```python
from build123d import *

# Parameters (mm, degrees)
SKETCH1_W                       = 160
SKETCH1_H                       = 36
BOSS_EXTRUDE1_DEPTH             = 3
SKETCH3_W                       = 160
SKETCH3_H                       = 36
SKETCH3_W_2                     = 156
SKETCH3_H_2                     = 32
BOSS_EXTRUDE3_DEPTH             = 20
SKETCH4_W                       = 2
SKETCH4_H                       = 1
CUT_EXTRUDE1_DEPTH              = 20
SKETCH5_R                       = 4.5
BOSS_EXTRUDE4_DEPTH             = 20
F_5_0MM_DOWEL_HOLE1_D           = 5
F_5_0MM_DOWEL_HOLE1_DEPTH       = 4.6
F_5_0MM_DOWEL_HOLE1_CSINK_D     = 6
F_5_0MM_DOWEL_HOLE1_CSINK_ANGLE = 90
FILLET3_R                       = 3
M5_CLEARANCE_HOLE2_D            = 5.5
FILLET4_R                       = 1
M5_CLEARANCE_HOLE3_D            = 5.5
M5_CLEARANCE_HOLE3_DEPTH        = 10
M5_CLEARANCE_HOLE3_TIP          = 1.652366702


with BuildPart() as part:
    # Sketch1 → Boss-Extrude1 (new body)
    with BuildSketch(Plane.XY):
        Rectangle(SKETCH1_W, SKETCH1_H)
    extrude(amount=BOSS_EXTRUDE1_DEPTH)

    # Sketch3 → Boss-Extrude3 (add)
    with BuildSketch(Plane.XY.offset(3)):
        Rectangle(SKETCH3_W, SKETCH3_H)
        Rectangle(SKETCH3_W_2, SKETCH3_H_2, mode=Mode.SUBTRACT)
    extrude(amount=BOSS_EXTRUDE3_DEPTH)

    # Sketch4 → Cut-Extrude1 (cut)
    with BuildSketch(Plane.XY.offset(23)):
        with Locations((79, 0)):
            Rectangle(SKETCH4_W, SKETCH4_H)
    cut_extrude1 = extrude(amount=-CUT_EXTRUDE1_DEPTH, mode=Mode.SUBTRACT)

    # Sketch5 → Boss-Extrude4 (add)
    with BuildSketch(Plane.XY.offset(3)):
        with Locations((75, 13)):
            Circle(SKETCH5_R)
        with Locations((75, -13)):
            Circle(SKETCH5_R)
    boss_extrude4 = extrude(amount=BOSS_EXTRUDE4_DEPTH)

    # Ø5.0mm Dowel Hole1
    with Locations(Plane.XY.offset(23)):
        with Locations((75, 13), (75, -13)):
            f_5_0mm_dowel_hole1 = CounterSinkHole(F_5_0MM_DOWEL_HOLE1_D / 2, F_5_0MM_DOWEL_HOLE1_CSINK_D / 2, depth=F_5_0MM_DOWEL_HOLE1_DEPTH, counter_sink_angle=F_5_0MM_DOWEL_HOLE1_CSINK_ANGLE)

    # Fillet3
    fillet3_edges = [part.edges().sort_by_distance(p)[0] for p in [
        (-80, 18, 11.5),
        (80, 18, 11.5),
        (80, -18, 11.5),
        (-80, -18, 11.5),
    ]]
    fillet(fillet3_edges, radius=FILLET3_R)

    # M5 Clearance Hole2 (through all)
    with Locations(Plane(origin=(0, 0, 0), x_dir=(-1, 0, 0), z_dir=(0, 0, -1))):
        with Locations((-70, 0), (70, 0)):
            m5_clearance_hole2 = Hole(M5_CLEARANCE_HOLE2_D / 2)

    # Mirror2: Cut-Extrude1, Boss-Extrude4, Ø5.0mm Dowel Hole1, M5 Clearance Hole2 across plane
    add(cut_extrude1.mirror(Plane(origin=(0, 0, 0), x_dir=(0, 0, 1), z_dir=(1, 0, 0))), mode=Mode.SUBTRACT)
    add(boss_extrude4.mirror(Plane(origin=(0, 0, 0), x_dir=(0, 0, 1), z_dir=(1, 0, 0))))
    add(f_5_0mm_dowel_hole1.mirror(Plane(origin=(0, 0, 0), x_dir=(0, 0, 1), z_dir=(1, 0, 0))), mode=Mode.SUBTRACT)
    add(m5_clearance_hole2.mirror(Plane(origin=(0, 0, 0), x_dir=(0, 0, 1), z_dir=(1, 0, 0))), mode=Mode.SUBTRACT)

    # Fillet4
    fillet4_edges = [part.edges().sort_by_distance(p)[0] for p in [
        (-78, -9.645898034, 13),
        (-78, -0.5, 13),
        (-80, -0.5, 13),
        (-80, 0.5, 13),
        (-78, 0.5, 13),
        (-78, 9.645898034, 13),
        (-71.645898034, 16, 13),
        (71.645898034, 16, 13),
        (78, 0.5, 13),
        (80, 0.5, 13),
        (80, -0.5, 13),
        (78, -0.5, 13),
        (78, -9.645898034, 13),
        (71.645898034, -16, 13),
        (-71.645898034, -16, 13),
        (78, 9.645898034, 13),
    ]]
    fillet(fillet4_edges, radius=FILLET4_R - 0.0001)  # a hair under: the kernel refuses the full size

    # M5 Clearance Hole3
    with Locations(Plane(origin=(80, 0, 0), x_dir=(0, 0, -1), z_dir=(1, 0, 0))):
        with Locations((-21.351359234, 0)):
            Hole(M5_CLEARANCE_HOLE3_D / 2, depth=M5_CLEARANCE_HOLE3_DEPTH)
            with Locations((0, 0, -(M5_CLEARANCE_HOLE3_DEPTH + M5_CLEARANCE_HOLE3_TIP / 2))):  # 118° drill point
                Cone(0, M5_CLEARANCE_HOLE3_D / 2, M5_CLEARANCE_HOLE3_TIP, mode=Mode.SUBTRACT)


solid = part.part
```
Verification items for the finished model (mm, model axes). A direction names the side the tool comes from. Round coordinates to 2 decimals unless told otherwise and drop trailing zeros. Order: outer loops, then holes, each group sorted by start corner. A loop starts at its lowest first (then second) coordinate and runs counter-clockwise, first axis right, second up. Notation, with made-up numbers: (-33.75, 66.25) -> (-12.75, 66.25) arc R20 cw to (-12.75, 70.25) -> close; hole circle Ø5 at (69.25, -30.5). An arc over 180 degrees is marked (long way). Put each result on its own line as item: value. Start each with the question number.
(1) Depth check by flat-ended pin: pin 1 Ø4.5 at (x, y) = (-70, 0) entering from -Z; pin 2 Ø2.5 at (x, y) = (75, -13.5) entering from +Z; pin 3 Ø1 at (x, y) = (12.5, -3.5) entering from +Z; pin 4 Ø2.5 at (x, y) = (74, 14) entering from +Z. Enter the tip coordinate at first touch or a pass-through.
(2) Material ranges on line 1 along X through (y, z) = (-13, 20.85); line 2 along X through (y, z) = (0, 1.6); line 3 along Y through (x, z) = (75, 21.15), recorded low to high.
(3) Section check A-A (x = -12.5). Enter the section's corners in (y, z).
(4) Tool access check on faces 1 (the face through (-80, -4, 11)), 2 (the face through (-71.87, -9.767, 12.86)). Record the directions out of +Z, -Z, +X, -X, +Y, -Y that give a thin tool (end or side, any length) a straight path to the whole face; none if there is none.
(5) Draft check along X on faces 3 (the face through (-78, -5, 13)), 4 (the face through (80, -4, 11)), 5 (the face through (-1, -18, 11)), 6 (the face through (78, -5, 13)). Enter one of: +X half, -X half, draft (parallel to the pull), parting line (faces both ways), or undercut.
(6) Section check C-C (x = 75). Enter the section's corners in (y, z), then the cut area to 4 significant figures.
(7) Section check B-B (y = -6). Enter the section's corners in (x, z).
Completed:
1. pin 1: passes through
1. pin 2: stops at z = 18.4
1. pin 3: stops at z = 3
1. pin 4: stops at z = 22.66
2. line 1: x = -80 to -77.5, -72.5 to -70.5, 70.5 to 72.5, 77.5 to 80
2. line 2: x = -80 to -72.75, -67.25 to 67.25, 72.75 to 80
2. line 3: y = -18 to -15.5, -10.5 to -8.5, 8.5 to 10.5, 15.5 to 18
3. outline: (-18, 0) -> (18, 0) -> (18, 23) -> (16, 23) -> (16, 3) -> (-16, 3) -> (-16, 23) -> (-18, 23) -> close
4. face 1: +Z, -Z, -X, +Y, -Y
4. face 2: +Z
5. face 3: undercut
5. face 4: +X half
5. face 5: draft
5. face 6: undercut
6. outline: (-18, 0) -> (18, 0) -> (18, 23) -> (16, 23) -> (15.5, 22.5) -> (15.5, 18.4) -> (10.5, 18.4) -> (10.5, 22.5) -> (10, 23) -> (8.5, 23) -> (8.5, 3) -> (-8.5, 3) -> (-8.5, 23) -> (-10, 23) -> (-10.5, 22.5) -> (-10.5, 18.4) -> (-15.5, 18.4) -> (-15.5, 22.5) -> (-16, 23) -> (-18, 23) -> close
6. area: 441.5 mm2
7. outline: (-80, 0) -> (80, 0) -> (80, 23) -> (78, 23) -> (78, 3) -> (-78, 3) -> (-78, 23) -> (-80, 23) -> close
